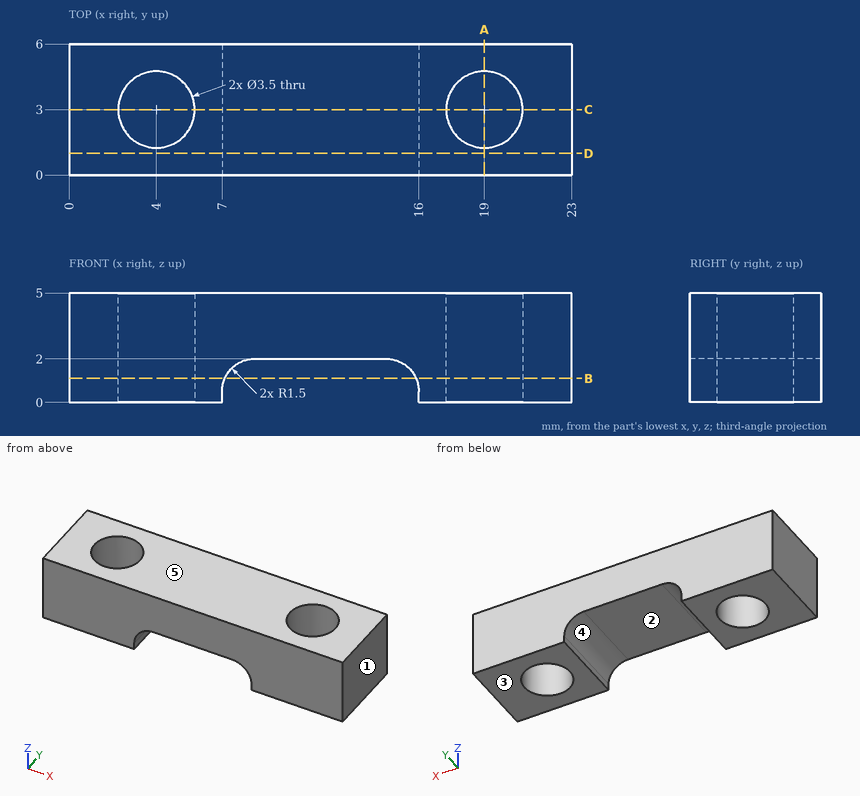
Source: three-view drawing plus pictorial views. Frame: mm from the lowest corner of the part. A direction names the side the tool comes from. Coordinates: 2 decimals unless noted, no trailing zeros. Order: outer loops, then holes, each group sorted by start corner. A loop starts at its lowest first (then second) coordinate and runs counter-clockwise, first axis right, second up. Notation, with made-up numbers: M 64.5,43 L 72.5,43 A17 cw 72.5,62 Z; hole C 77,21.25 d7. An arc over 180 degrees is marked long. Answer in a Markdown table with one row per item.
(1) Access query for the marked faces 4 and 5. Directions: +Z, -Z, +X, -X, +Y, -Y. A direction counts if a zero-diameter tool reaches every point of the face in a straight line with its end or side. Return the directions, or none.
Numbers:
| item | result |
|---|---|
| face 4 | -Z, +Y, -Y |
| face 5 | +Z, +X, -X, +Y, -Y |
(2) Section query B-B, the plane z = 1.1. Output: boundary loops of the cut face in (x, y), plus the area to 3 significant figures.
Numbers:
| item | result |
|---|---|
| outline | M 0,0 L 7.13,0 L 7.13,6 L 0,6 Z; M 15.87,0 L 23,0 L 23,6 L 15.87,6 Z; hole C 4,3 d3.5; hole C 19,3 d3.5 |
| area | 66.3 mm^2 |
(3) Section query C-C, the plane y = 3. Output: boundary loops of the cut face in (x, z), plus the area to 3 significant figures.
Numbers:
| item | result |
|---|---|
| outline | M 0,0 L 2.25,0 L 2.25,5 L 0,5 Z; M 5.75,0 L 7,0 L 7,0.5 A1.5 cw 8.5,2 L 14.5,2 A1.5 cw 16,0.5 L 16,0 L 17.25,0 L 17.25,5 L 5.75,5 Z; M 20.75,0 L 23,0 L 23,5 L 20.75,5 Z |
| area | 63.0 mm^2 |
(4) Material intervals for line 1 (Y direction, x = 4, z = 2.6); line 2 (X direction, y = 1.75, z = 1.4); line 3 (X direction, y = 2.35, z = 4.4), sorted ascending. Write a range as [from, to].
Numbers:
| item | result |
|---|---|
| line 1 | y = [0, 1.25], [4.75, 6] |
| line 2 | x = [0, 2.78], [5.22, 7.3], [15.7, 17.78], [20.22, 23] |
| line 3 | x = [0, 2.38], [5.62, 17.38], [20.62, 23] |
(5) Section query D-D, the plane y = 1. Output: boundary loops of the cut face in (x, z), plus the area to 3 significant figures.
Numbers:
| item | result |
|---|---|
| outline | M 0,0 L 7,0 L 7,0.5 A1.5 cw 8.5,2 L 14.5,2 A1.5 cw 16,0.5 L 16,0 L 23,0 L 23,5 L 0,5 Z |
| area | 98.0 mm^2 |
(6) Draft query along X for the marked faces 1, 2 and 3. Return one class per face: pulls with the +X half, pulls with the -X half, needs draft (parallel to the pull), parting line crosses it, or undercut.
Numbers:
| item | result |
|---|---|
| face 1 | pulls with the +X half |
| face 2 | undercut |
| face 3 | needs draft |
(7) Contact query for flat-ended pins moving along their axis: pin 1 Ø2 at (x, y) = (4, 3) entering from +Z; pin 2 Ø3 at (y, z) = (2.5, 1.5) entering from -X; pin 3 Ø2 at (x, y) = (14, 5) entering from -Z. Output: stop coordinate, or through.
Numbers:
| item | result |
|---|---|
| pin 1 | passes through |
| pin 2 | stops at x = 0 |
| pin 3 | stops at z = 1.91 |
(8) Section query A-A, the plane x = 19. Output: boundary loops of the cut face in (y, z), plus the area to 3 significant figures.
Numbers:
| item | result |
|---|---|
| outline | M 0,0 L 1.25,0 L 1.25,5 L 0,5 Z; M 4.75,0 L 6,0 L 6,5 L 4.75,5 Z |
| area | 12.5 mm^2 |
